Autodesk Inventor part; units mm, degrees
ref_plane "YZ Plane" through (0, 0, 0) normal (1, 0, 0) x (0, 1, 0)
ref_plane "XZ Plane" through (0, 0, 0) normal (0, 1, 0) x (-1, 0, 0)
ref_plane "XY Plane" through (0, 0, 0) normal (0, 0, 1) x (1, 0, 0)
sketch "Sketch1" plane through (0, 0, 0) normal (0, 1, 0) x (-1, 0, 0)
  line L0 (-15, -15) -> (15, -15)
  line L1 (15, -15) -> (15, 15)
  line L2 (15, 15) -> (-15, 15)
  line L3 (-15, 15) -> (-15, -15)
  line L4 (-15, -15) -> (15, 15) construction
  line L5 (15, -15) -> (-15, 15) construction
  point P0 (0, 0)
  dimension "d7" = 30
  dimension "d8" = 30
extrude "Base plate" add sketch "Sketch1" along normal blind 3
sketch "Sketch5" plane through (0, 3, 0) normal (0, 1, 0) x (1, 0, 0)
  circle A0 centre (0, 0) radius 9.5
  line L0 (-15, 15) -> (-15, -15)
  line L1 (-15, -15) -> (15, -15)
  line L2 (15, 15) -> (-15, 15)
  point P0 (0, 0)
  point P1 (8.0777, -15)
  point P2 (-8.0777, -15)
  dimension "d19" = 19
  dimension "d20" = 15
  dimension "d21" = 15
extrude "Sleutel 19" cut sketch "Sketch5" against normal through all
sketch "Sketch9" plane through (0, 3, 0) normal (0, 1, 0) x (1, 0, 0)
  line L0 (-9.3784, 15) -> (9.5, 15)
  line L1 (9.5, 15) -> (9.5, 8)
  line L2 (9.5, 8) -> (-9.3784, 8)
  line L3 (-9.3784, 8) -> (-9.3784, 15)
  circle A0 centre (0, 0) radius 9.5
  line L4 (15, 15) -> (-15, 15)
  point P0 (0, 0)
  point P1 (-5.1235, 8)
  point P2 (5.1235, 8)
  point P3 (-8.0777, 15)
  point P4 (8.0777, 15)
  dimension "d33" = 8
  dimension "d34" = 0
extrude "Extrusion7" add sketch "Sketch9" against normal up to surface (3 mm away) contours L0 L1 L2 A0 L3 | A0 L2 picked at (-1.0613, 8.3168)
sketch "Sketch10" plane through (0, 3, 0) normal (0, 1, 0) x (1, 0, 0)
  line L0 (-10.3172, -11) -> (10, -11)
  line L1 (10, -11) -> (10, -8)
  line L2 (10, -8) -> (-10.3172, -8)
  line L3 (-10.3172, -8) -> (-10.3172, -11)
  arc A0 (-5.1235, 8) -> (5.1235, 8) centre (0, 0) ccw
  point P0 (0, 0)
  point P1 (5.1235, -8)
  point P2 (-5.1235, -8)
  point P3 (-8.0777, 15)
  point P4 (8.0777, 15)
  dimension "d37" = 8
extrude "Extrusion8" add sketch "Sketch10" against normal up to surface (3 mm away)
properties part number "Holes_Test2"
Could you check a few things on this model? Use its own coordinates, in mm. A direction names the side the tool comes from. Give positions to 0.01 mm unless a question says otherwise; leave off trailing zeros. Write each loop counter-clockwise with the first axis right and the second up, starting at its lowest first coordinate (ties: lowest second). Pieces come first, ordered by that corner, then holes. Notation, with made-up numbers: (52.5, -1.5) - (88.5, -1.5) arc R15 ccw to (88.5, 15.5) - close; hole circle Ø10 at (-14, -9.5). An arc over 180 degrees is marked (long way). Use CSV: the item, a comma, the result in double quotes. Start each with the question number.
Item 1: I want a section at B-B, the plane x = 0. Please give me the cut outline in (y, z), then the cut area to 3 significant figures.
Item 2: If we mould it in two halves opening along X, with no side actions, what happens to faces 1 (the face through (0, 1, 15)), 2 (the face through (0, 2, 8)), 3 (the face through (15, 1, 0))? For each: pulls with the +X half, pulls with the -X half, needs draft (parallel to the pull), parting line crosses it, or undercut.
Item 3: If I drill on line 1 along Z through (x, y) = (2.25, 2.7); line 2 along X through (y, z) = (2.7, 5.75); line 3 along X through (y, z) = (2.2, 6), over which ranges is the centre line in solid material (lowest first)?
Item 4: I want a section at C-C, the plane z = 1.75. Please give me the cut outline in (x, y), then the cut area to 3 significant figures.
Item 5: I want a section at A-A, the plane y = 1.8. Please give me the cut outline in (x, z), then the cut area to 3 significant figures.
Item 6: For faces 4 (the face through (-9.5, 1.5, -0.1)), 5 (the face through (-15, 1, 0)), which set-ups out of +Z, -Z, +X, -X, +Y, -Y let a thin tool reach every point of the face, with its end or its side?
Findings:
1,outline,"(0, -15) - (3, -15) - (3, -8) - (0, -8) - close; (0, 8) - (3, 8) - (3, 15) - (0, 15) - close"
1,area,"42.0 mm2"
2,face 1,"needs draft"
2,face 2,"undercut"
2,face 3,"pulls with the +X half"
3,line 1,"z = -15 to -8, 8 to 15"
3,line 2,"x = -15 to -7.56, 7.56 to 15"
3,line 3,"x = -15 to -7.37, 7.37 to 15"
4,outline,"(-15, 0) - (-9.34, 0) - (-9.34, 3) - (-15, 3) - close; (9.34, 0) - (15, 0) - (15, 3) - (9.34, 3) - close"
4,area,"34.0 mm2"
5,outline,"(-15, -15) - (15, -15) - (15, 15) - (-15, 15) - close; hole (-5.12, -8) - (5.12, -8) arc R9.5 ccw to (5.12, 8) - (-5.12, 8) arc R9.5 ccw to start"
5,area,"637 mm2"
6,face 4,"+Y, -Y"
6,face 5,"+Z, -Z, -X, +Y, -Y"
